```python
from build123d import *

# Parameters (mm, degrees)
SKETCH1_W           = 121
SKETCH1_H           = 60
SKETCH1_R           = 5
SKETCH1_R_2         = 1.25
SKETCH1_W_2         = 8
SKETCH1_H_2         = 4
BOSS_EXTRUDE1_DEPTH = 4


with BuildPart() as part:
    # Sketch1 → Boss-Extrude1 (new body)
    with BuildSketch(Plane.XY):
        with Locations((-18.5, 11.603893248)):
            Rectangle(SKETCH1_W, SKETCH1_H)
        with Locations((-34, 11.603893248)):
            Circle(SKETCH1_R, mode=Mode.SUBTRACT)
        with Locations((0, 11.603893248)):
            Circle(SKETCH1_R, mode=Mode.SUBTRACT)
        with Locations((28, -12.396106752)):
            Circle(SKETCH1_R_2, mode=Mode.SUBTRACT)
        with Locations((-60, -1.396106752)):
            Rectangle(SKETCH1_W_2, SKETCH1_H_2, mode=Mode.SUBTRACT)
    extrude(amount=BOSS_EXTRUDE1_DEPTH)


solid = part.part
```
The model under review builds one solid part; all positions refer to its coordinate system, in mm. A direction names the side the tool comes from. Give positions to 0.01 mm unless a question says otherwise; leave off trailing zeros. Order: outer loops, then holes, each group sorted by start corner. A loop starts at its lowest first (then second) coordinate and runs counter-clockwise, first axis right, second up. Notation, with made-up numbers: (26, 82) - (38, 82) arc R15 cw to (38, 96) - close; hole circle Ø9 at (57, 9). An arc over 180 degrees is marked (long way). Use CSV: the item, a comma, the result in double quotes. Start each with the question number.
Q1. Clearance check with flat-ended pins moving along their axes: pin 1 Ø13 at (x, y) = (0, 11.6) entering from +Z; pin 2 Ø1.5 at (x, y) = (28, -12.4) entering from +Z. State where each tip first meets the part, or that it passes through.
Q2. To check wall thickness, follow line 1 along Y through (x, z) = (28, 2.7); line 2 along X through (y, z) = (12, 2.8); line 3 along X through (y, z) = (8, 2.15). State the ranges of each line that lie inside material, in increasing order. Write a range as [from, to].
Q3. We need section B-B, the plane z = 1.45. Write out the cut boundary in (x, y), and give its area (3 significant figures).
Q4. We need section C-C, the plane x = -34. Write out the cut boundary in (y, z), and give its area (3 significant figures).
Q5. Tool access review of faces 1 (the flat face through (-64, -1, 2)), 2 (the flat face through (-79, 11, 2)): name each direction out of +Z, -Z, +X, -X, +Y, -Y from which nothing blocks a thin tool from reaching the whole face with its end or side.
Q6. The part is to be moulded in two halves that separate along Y. For faces 3 (the flat face through (42, 11, 2)), 4 (the flat face through (-19, -18.396, 2)), 5 (the flat face through (-60, 0.604, 2)), say which applies: +Y half, -Y half, draft (parallel to the pull), parting line (faces both ways), or undercut.
Q7. We need section A-A, the plane x = 28. Write out the cut boundary in (y, z).
Outcome:
1,pin 1,"stops at z = 4"
1,pin 2,"passes through"
2,line 1,"y = [-18.4, -13.65], [-11.15, 41.6]"
2,line 2,"x = [-79, -38.98], [-29.02, -4.98], [4.98, 42]"
2,line 3,"x = [-79, -37.47], [-30.53, -3.47], [3.47, 42]"
3,outline,"(-79, -18.4) - (42, -18.4) - (42, 41.6) - (-79, 41.6) - close; hole (-64, -3.4) - (-56, -3.4) - (-56, 0.6) - (-64, 0.6) - close; hole circle Ø10 at (-34, 11.6); hole circle Ø10 at (0, 11.6); hole circle Ø2.5 at (28, -12.4)"
3,area,"7,070 mm^2"
4,outline,"(-18.4, 0) - (6.6, 0) - (6.6, 4) - (-18.4, 4) - close; (16.6, 0) - (41.6, 0) - (41.6, 4) - (16.6, 4) - close"
4,area,"200 mm^2"
5,face 1,"+Z, -Z"
5,face 2,"+Z, -Z, -X, +Y, -Y"
6,face 3,"draft"
6,face 4,"-Y half"
6,face 5,"undercut"
7,outline,"(-18.4, 0) - (-13.65, 0) - (-13.65, 4) - (-18.4, 4) - close; (-11.15, 0) - (41.6, 0) - (41.6, 4) - (-11.15, 4) - close"
